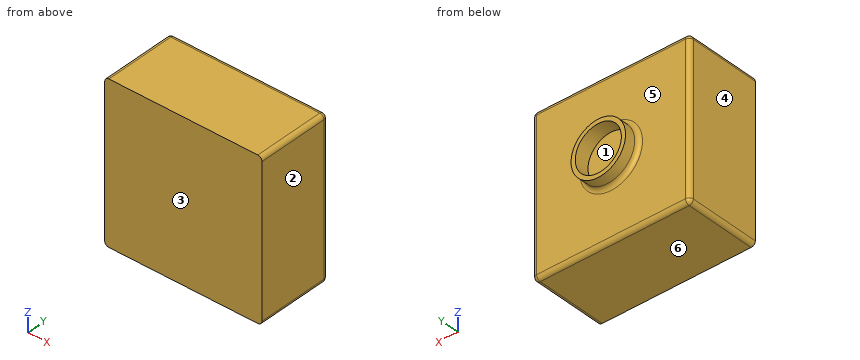
```python
from build123d import *

# Parameters (mm, degrees)
SKETCH1_W           = 375
SKETCH1_H           = 375
BOSS_EXTRUDE1_DEPTH = 180
SKETCH2_R           = 65
BOSS_EXTRUDE2_DEPTH = 35
SKETCH3_R           = 55
CUT_EXTRUDE1_DEPTH  = 35
FILLET1_R           = 10
FILLET2_R           = 10


with BuildPart() as part:
    # Sketch1 → Boss-Extrude1 (new body)
    with BuildSketch(Plane(origin=(0, 0, 0), x_dir=(1, 0, 0), z_dir=(0, 1, 0))):
        Rectangle(SKETCH1_W, SKETCH1_H)
    extrude(amount=BOSS_EXTRUDE1_DEPTH)

    # Sketch2 → Boss-Extrude2 (add)
    with BuildSketch(Plane(origin=(0, 180, 0), x_dir=(1, 0, 0), z_dir=(0, 1, 0))):
        with Locations(Location((0, 0, 0), (0, 0, 270))):
            Circle(SKETCH2_R)
    extrude(amount=BOSS_EXTRUDE2_DEPTH)

    # Sketch3 → Cut-Extrude1 (cut)
    with BuildSketch(Plane(origin=(0, 215, 0), x_dir=(1, 0, 0), z_dir=(0, 1, 0))):
        with Locations(Location((0, 0, 0), (0, 0, 270))):
            Circle(SKETCH3_R)
    extrude(amount=-CUT_EXTRUDE1_DEPTH, mode=Mode.SUBTRACT)

    # Fillet1
    fillet1_edges = [part.edges().sort_by_distance(p)[0] for p in [
        (0, 180, -65),
    ]]
    fillet(fillet1_edges, radius=FILLET1_R)

    # Fillet2
    fillet2_edges = [part.edges().sort_by_distance(p)[0] for p in [
        (187.5, 180, 0),
        (0, 180, -187.5),
        (-187.5, 180, 0),
        (-187.5, 90, -187.5),
        (187.5, 90, -187.5),
        (187.5, 90, 187.5),
        (-187.5, 90, 187.5),
        (0, 180, 187.5),
    ]]
    fillet(fillet2_edges, radius=FILLET2_R)


solid = part.part
```
Build history of the part. All positions in model axes, mm. Face numbers are marked on the shaded views. A direction names the side the tool comes from. Round coordinates to 2 decimals unless told otherwise and drop trailing zeros. Order: outer loops, then holes, each group sorted by start corner. A loop starts at its lowest first (then second) coordinate and runs counter-clockwise, first axis right, second up. Notation, with made-up numbers: (-4.5, -7.5) - (36.5, -7.5) arc R21 cw to (36.5, 31.5) - close; hole circle Ø7 at (62, -19.5). An arc over 180 degrees is marked (long way). Use a Markdown table: item, result.
1) Tool access for the marked faces 5 and 6: list every direction of +Z, -Z, +X, -X, +Y, -Y with a clear straight run to the whole face (end or side of a thin tool).
Recorded:
| item | result |
|---|---|
| face 5 | +Y |
| face 6 | -Z, +X, -X, +Y, -Y |
2) Saw through at A-A on z = 0. Write the cut outline in (x, y).
Recorded:
| item | result |
|---|---|
| outline | (-187.5, 0) - (187.5, 0) - (187.5, 170) arc R10 ccw to (177.5, 180) - (75, 180) arc R10 cw to (65, 190) - (65, 215) - (55, 215) - (55, 180) - (-55, 180) - (-55, 215) - (-65, 215) - (-65, 190) arc R10 cw to (-75, 180) - (-177.5, 180) arc R10 ccw to (-187.5, 170) - close |
3) Saw through at D-D on z = 112. Write the cut outline in (x, y), and give its area (3 significant figures).
Recorded:
| item | result |
|---|---|
| outline | (-187.5, 0) - (187.5, 0) - (187.5, 170) arc R10 ccw to (177.5, 180) - (-177.5, 180) arc R10 ccw to (-187.5, 170) - close |
| area | 67,500 mm² |
4) Pull direction X, two halves, no side cores. Call the marked faces 1, 2, 3 and 4: pulls with the +X half, pulls with the -X half, needs draft (parallel to the pull), parting line crosses it, or undercut.
Recorded:
| item | result |
|---|---|
| face 1 | undercut |
| face 2 | pulls with the +X half |
| face 3 | needs draft |
| face 4 | pulls with the -X half |
5) Wall check: L1, parallel to X at y = 204, z = 0; L2, parallel to Y at x = -153, z = 129; L3, parallel to X at y = 202.5, z = -44. Give the ranges that are in metal, low to high.
Recorded:
| item | result |
|---|---|
| L1 | x = -65 to -55, 55 to 65 |
| L2 | y = 0 to 180 |
| L3 | x = -47.84 to -33, 33 to 47.84 |
6) Saw through at B-B on x = 92.5. Write the cut outline in (y, z), and give its area (3 significant figures).
Recorded:
| item | result |
|---|---|
| outline | (0, -187.5) - (170, -187.5) arc R10 ccw to (180, -177.5) - (180, 177.5) arc R10 ccw to (170, 187.5) - (0, 187.5) - close |
| area | 67,500 mm² |
7) Flat gauge pins, fed straight in: pin 1 Ø10 at (y, z) = (176.5, 126) entering from -X; pin 2 Ø2 at (x, z) = (-67.5, 126.5) entering from +Y. Where does each tip first touch, or does it go through?
Recorded:
| item | result |
|---|---|
| pin 1 | stops at x = -187.39 |
| pin 2 | stops at y = 180 |
8) Saw through at C-C on y = 195. Write the cut outline in (x, z).
Recorded:
| item | result |
|---|---|
| outline | circle Ø130 at (0, 0); hole circle Ø110 at (0, 0) |
